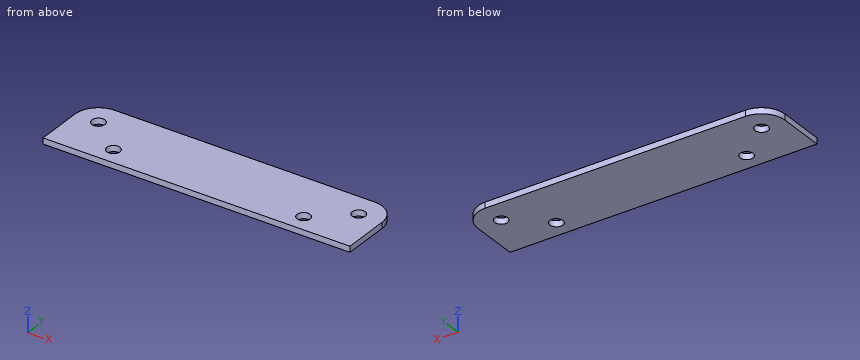
```python
from build123d import *

# Parameters (mm, degrees)
SKETCH1_W                   = 167.005
SKETCH1_H                   = 38.1
BOSS_EXTRUDE1_DEPTH         = 3.175
FILLET1_R                   = 12.7
F_1_4_CLEARANCE_HOLE1_D     = 7.14248
F_1_4_CLEARANCE_HOLE1_DEPTH = 3.175


with BuildPart() as part:
    # Sketch1 → Boss-Extrude1 (new body)
    with BuildSketch(Plane.XY):
        with Locations((0, -1694.09345438)):
            Rectangle(SKETCH1_W, SKETCH1_H)
    extrude(amount=BOSS_EXTRUDE1_DEPTH)

    # Fillet1
    fillet1_edges = [part.edges().sort_by_distance(p)[0] for p in [
        (-83.5025, -1675.04345438, 1.5875),
        (83.5025, -1675.04345438, 1.5875),
    ]]
    fillet(fillet1_edges, radius=FILLET1_R)

    # 1/4 Clearance Hole1
    with Locations(Plane.XY.offset(3.175)):
        with Locations((-70.8025, -1687.74345438), (70.8025, -1687.74345438), (51.7525, -1703.61845438), (-51.7525, -1703.61845438)):
            Hole(F_1_4_CLEARANCE_HOLE1_D / 2, depth=F_1_4_CLEARANCE_HOLE1_DEPTH)


solid = part.part
```
Could you check a few things on this model? Use its own coordinates, in mm. Give positions to 0.01 mm unless a question says otherwise; leave off trailing zeros. Loops run counter-clockwise (first coordinate to the right, second up) from the corner with the lowest first, then second, coordinate; pieces in that order, holes last. Notation, with made-up numbers: (-11.75, 18.25) - (-3.75, 18.25) arc R6 cw to (-3.75, 23.25) - close; hole circle Ø2 at (13, 31.25). An arc over 180 degrees is marked (long way). Answer in a Markdown table with one row per item. Add a question column.
Q1. Please list where these lines run through material, in increasing order: L1, parallel to X at y = -1688, z = 1.9; L2, parallel to X at y = -1690.5, z = 1.15; L3, parallel to Y at x = 51, z = 3. Write a range as from..to.
Q2. If we section it at A-A (y = -1701.5): List the corners of the cut face in (x, z) for me (1 decimal).
Q3. If we section it at B-B (z = 2.65): List the corners of the cut face in (x, y) for me.
Q4. If we section it at C-C (y = -1678): List the corners of the cut face in (x, z) for me (3 decimals), plus the area to 3 significant figures.
The answers:
| question | item | result |
|---|---|---|
| 1 | L1 | x = -83.5..-74.36, -67.24..67.24, 74.36..83.5 |
| 1 | L2 | x = -83.5..-73.07, -68.53..68.53, 73.07..83.5 |
| 1 | L3 | y = -1713.14..-1707.11, -1700.13..-1675.04 |
| 2 | outline | (-83.5, 0) - (-54.6, 0) - (-54.6, 3.2) - (-83.5, 3.2) - close; (-48.9, 0) - (48.9, 0) - (48.9, 3.2) - (-48.9, 3.2) - close; (54.6, 0) - (83.5, 0) - (83.5, 3.2) - (54.6, 3.2) - close |
| 3 | outline | (-83.5, -1713.14) - (83.5, -1713.14) - (83.5, -1687.74) arc R12.7 ccw to (70.8, -1675.04) - (-70.8, -1675.04) arc R12.7 ccw to (-83.5, -1687.74) - close; hole circle Ø7.14 at (-70.8, -1687.74); hole circle Ø7.14 at (-51.75, -1703.62); hole circle Ø7.14 at (51.75, -1703.62); hole circle Ø7.14 at (70.8, -1687.74) |
| 4 | outline | (-78.948, 0) - (78.948, 0) - (78.948, 3.175) - (-78.948, 3.175) - close |
| 4 | area | 501 mm^2 |
